Geometry check sheet. Reference: the model listing, model coordinates, mm. A direction names the side the tool comes from. Round coordinates to 2 decimals unless told otherwise and drop trailing zeros. Write each loop counter-clockwise with the first axis right and the second up, starting at its lowest first coordinate (ties: lowest second). Pieces come first, ordered by that corner, then holes. Notation, with made-up numbers: (-34, 71) - (-8, 71) arc R25 cw to (-8, 109) - close; hole circle Ø3 at (20, 36.25). An arc over 180 degrees is marked (long way). Return JSON: item names as keys, results as strings.
```python
from build123d import *

# Parameters (mm, degrees)
F0_R     = 0.8
F1_DEPTH = 3
F2_R     = 0.8
F3_DEPTH = 39.501
F4_R     = 1


with BuildPart() as f1:
    # F0 (on Top) → F1 (new body)
    with BuildSketch(Plane.XY):
        with BuildLine():
            Line((13.5, 19.75), (-13.5, 19.75))
            ThreePointArc((-13.5, 19.75), (-14.56066, 19.31066), (-15, 18.25))
            Line((-15, 18.25), (-15, -18.25))
            ThreePointArc((-15, -18.25), (-14.56066, -19.31066), (-13.5, -19.75))
            Line((-13.5, -19.75), (13.5, -19.75))
            ThreePointArc((13.5, -19.75), (14.56066, -19.31066), (15, -18.25))
            Line((15, -18.25), (15, 18.25))
            ThreePointArc((15, 18.25), (14.56066, 19.31066), (13.5, 19.75))
        make_face()
        with Locations((-10, -10)):
            Circle(F0_R, mode=Mode.SUBTRACT)
        with Locations((10, -10)):
            Circle(F0_R, mode=Mode.SUBTRACT)
        with Locations((-10, 10)):
            Circle(F0_R, mode=Mode.SUBTRACT)
        with BuildLine():
            ThreePointArc((1.25, 9.921567), (7.5, 6.614378), (10, 0))
            ThreePointArc((10, 0), (7.5, -6.614378), (1.25, -9.921567))
            Line((1.25, -9.921567), (1.25, -10))
            ThreePointArc((1.25, -10), (0, -11.25), (-1.25, -10))
            Line((-1.25, -10), (-1.25, -9.921567))
            ThreePointArc((-1.25, -9.921567), (-10, 0), (-1.25, 9.921567))
            Line((-1.25, 9.921567), (-1.25, 10))
            ThreePointArc((-1.25, 10), (0, 11.25), (1.25, 10))
            Line((1.25, 10), (1.25, 9.921567))
        make_face(mode=Mode.SUBTRACT)
        with Locations((10, 10)):
            Circle(F0_R, mode=Mode.SUBTRACT)
    extrude(amount=F1_DEPTH)

    # F2 (on face) → F3 (cut, through all)
    with BuildSketch(Plane.XZ.offset(19.75)):
        with Locations((0, 1.5)):
            Circle(F2_R)
        with Locations((10, 1.5)):
            Circle(F2_R)
        with Locations((-10, 1.5)):
            Circle(F2_R)
    extrude(amount=-F3_DEPTH, mode=Mode.SUBTRACT)

    # F4
    f4_edges = [f1.edges().sort_by_distance(p)[0] for p in [
        (1.25, 9.921567, 1.5),
        (-1.25, 9.921567, 1.5),
        (-1.25, -9.921567, 1.5),
        (1.25, -9.921567, 1.5),
    ]]
    fillet(f4_edges, radius=F4_R)


solid = f1.part
```
(1) Section check B-B, the plane y = 5. Enter the section's corners in (x, z), plus the area to 3 significant figures.
Response values:
{"outline": "(-15, 0) - (-8.66, 0) - (-8.66, 3) - (-15, 3) - close; (8.66, 0) - (15, 0) - (15, 3) - (8.66, 3) - close; hole circle Ø1.6 at (-10, 1.5); hole circle Ø1.6 at (10, 1.5)", "area": "34.0 mm^2"}
(2) Access from +Z, -Z, +X, -X, +Y, -Y to the whole of each face (thin tool, end or side, straight path). Record for faces 1 (the face through (0.916, -10.85, 1.479)), 2 (the face through (-0.17, 15.29, 0.72)).
Response values:
{"face 1": "+Z, -Z", "face 2": "+Y, -Y"}
(3) Release check for a two-part mould opening along X. For faces 3 (the face through (-15, 0, 1)), 4 (the face through (-10.2, 0.3, 0)), 5 (the face through (10.739, -0.14, 1.194)) record: pulls with the +X half, pulls with the -X half, needs draft (parallel to the pull), parting line crosses it, or undercut.
Response values:
{"face 3": "pulls with the -X half", "face 4": "needs draft", "face 5": "undercut"}
(4) Gauge pin test, flat ends, axial feed: pin 1 (1.8 mm diameter, centred on x = 10, z = 1.5, fed in from -Y); pin 2 (1.3 mm diameter, centred on x = -10, z = 1.5, fed in from +Y). Record the tip position at first contact, or that the pin passes through.
Response values:
{"pin 1": "stops at y = -19.75", "pin 2": "passes through"}
(5) Section check D-D, the plane z = 1.1. Give the number of separate pieces and of enclosed holes in the cut face, plus the area to 3 significant figures.
Response values:
{"separate pieces": "6", "enclosed holes": "0", "area": "737 mm^2"}
(6) Material ranges on line 1 along X through (y, z) = (16.5, 1.5); line 2 along X through (y, z) = (-5.5, 1.4); line 3 along Z through (x, y) = (-10, -3), recorded low to high. Write a range as [from, to].
Response values:
{"line 1": "x = [-15, -10.8], [-9.2, -0.8], [0.8, 9.2], [10.8, 15]", "line 2": "x = [-15, -10.79], [-9.21, -8.35], [8.35, 9.21], [10.79, 15]", "line 3": "z = [0, 0.7], [2.3, 3]"}
(7) Section check A-A, the plane x = 0. Enter the section's corners in (y, z), plus the area to 3 significant figures.
Response values:
{"outline": "(-19.75, 0) - (-11.25, 0) - (-11.25, 0.7) - (-19.75, 0.7) - close; (-19.75, 2.3) - (-11.25, 2.3) - (-11.25, 3) - (-19.75, 3) - close; (11.25, 0) - (19.75, 0) - (19.75, 0.7) - (11.25, 0.7) - close; (11.25, 2.3) - (19.75, 2.3) - (19.75, 3) - (11.25, 3) - close", "area": "23.8 mm^2"}
(8) Section check C-C, the plane x = -7. Enter the section's corners in (y, z), plus the area to 3 significant figures.
Response values:
{"outline": "(-19.75, 0) - (-7.14, 0) - (-7.14, 3) - (-19.75, 3) - close; (7.14, 0) - (19.75, 0) - (19.75, 3) - (7.14, 3) - close", "area": "75.7 mm^2"}
